Geometry check sheet. Reference: the model listing, model coordinates, mm. A direction names the side the tool comes from. Give positions to 0.01 mm unless a question says otherwise; leave off trailing zeros. Order: outer loops, then holes, each group sorted by start corner. A loop starts at its lowest first (then second) coordinate and runs counter-clockwise, first axis right, second up. Notation, with made-up numbers: M 39,3.25 L 70,3.25 A23 ccw 70,12.25 Z; hole C 5,15.5 d9. An arc over 180 degrees is marked long. Answer as CSV lines item,"result". Start each with the question number.
```python
from build123d import *

# Parameters (mm, degrees)
ESBO_O1_R                = 1.5
ESBO_O1_W                = 15
ESBO_O1_H                = 4
ESBO_O1_W_2              = 5
ESBO_O1_H_2              = 12
RESSALTO_EXTRUS_O1_DEPTH = 5
ESBO_O1_3_W              = 5
ESBO_O1_3_H              = 12
ESBO_O1_3_W_2            = 15
ESBO_O1_3_H_2            = 4
CORTE_EXTRUS_O1_DEPTH    = 2
RESSALTO_EXTRUS_O2_DEPTH = 10
ESBO_O3_R                = 1.5
CORTE_EXTRUS_O2_DEPTH    = 10


with BuildPart() as part:
    # Esbo_o1 → Ressalto-extrus_o1 (new body)
    with BuildSketch(Plane.XY):
        with BuildLine():
            ThreePointArc((40, 3), (39.121320344, 0.878679656), (37, 0))
            Line((37, 0), (0, 0))
            Line((0, 0), (0, 13))
            ThreePointArc((0, 13), (0.878679656, 15.121320344), (3, 16))
            Line((3, 16), (40, 16))
            Line((40, 16), (40, 3))
        make_face()
        with Locations((38, 14)):
            Circle(ESBO_O1_R, mode=Mode.SUBTRACT)
        with Locations((19, 14)):
            Circle(ESBO_O1_R, mode=Mode.SUBTRACT)
        with Locations((28.5, 8)):
            Rectangle(ESBO_O1_W, ESBO_O1_H, mode=Mode.SUBTRACT)
        with Locations((13, 8)):
            Rectangle(ESBO_O1_W_2, ESBO_O1_H_2, mode=Mode.SUBTRACT)
        with Locations((13, 8)):
            Rectangle(ESBO_O1_W_2, ESBO_O1_H_2)
        with Locations((28.5, 8)):
            Rectangle(ESBO_O1_W, ESBO_O1_H)
    extrude(amount=-RESSALTO_EXTRUS_O1_DEPTH)

    # Esbo_o1_3 → Corte-extrus_o1 (cut)
    with BuildSketch(Plane.XY):
        with Locations((13, 8)):
            Rectangle(ESBO_O1_3_W, ESBO_O1_3_H)
        with Locations((28.5, 8)):
            Rectangle(ESBO_O1_3_W_2, ESBO_O1_3_H_2)
    extrude(amount=-CORTE_EXTRUS_O1_DEPTH, mode=Mode.SUBTRACT)

    # Esbo_o2 → Ressalto-extrus_o2 (add)
    with BuildSketch(Plane.XZ):
        with BuildLine():
            Line((19.1, -5), (12.000000019, -5))
            ThreePointArc((12.000000019, -5), (17.086118989, -9.723976561), (12.75, -15.144551516))
            Line((12.75, -15.144551516), (12.75, -21.64580018))
            Line((12.75, -21.64580018), (14.75, -21.64580018))
            Line((14.75, -21.64580018), (14.75, -16.64580018))
            ThreePointArc((14.75, -16.64580018), (17.913332394, -14.029694645), (19.1, -10.1))
            Line((19.1, -10.1), (19.1, -5))
        make_face()
        with BuildLine():
            Line((12.000000019, -5), (4.9, -5))
            Line((4.9, -5), (4.9, -10.1))
            ThreePointArc((4.9, -10.1), (6.086667606, -14.029694645), (9.25, -16.64580018))
            Line((9.25, -16.64580018), (9.25, -21.64580018))
            Line((9.25, -21.64580018), (11.25, -21.64580018))
            Line((11.25, -21.64580018), (11.25, -15.144551516))
            ThreePointArc((11.25, -15.144551516), (6.913881012, -9.723976542), (12.000000019, -5))
        make_face()
    extrude(amount=-RESSALTO_EXTRUS_O2_DEPTH)

    # Esbo_o3 → Corte-extrus_o2 (cut)
    with BuildSketch(Plane(origin=(14.75, 0, 0), x_dir=(0, 0, -1), z_dir=(1, 0, 0))):
        with Locations((19.14580018, 5)):
            Circle(ESBO_O3_R)
    extrude(amount=-CORTE_EXTRUS_O2_DEPTH, mode=Mode.SUBTRACT)


solid = part.part
```
Item 1: Section check C-C on x = 7.5. Record the boundary of the cut face in (y, z).
Item 2: Draft check along Y on faces 5 (the face through (28, 10, -1)), 6 (the face through (36, 8, -1)), 7 (the face through (0, 6, -2)), 8 (the face through (39.14, 0.9, -2.46)). Enter one of: pulls with the +Y half, pulls with the -Y half, needs draft (parallel to the pull), parting line crosses it, or undercut.
Item 3: Access from +Z, -Z, +X, -X, +Y, -Y to the whole of each face (thin tool, end or side, straight path). Record for faces 1 (the face through (4.9, 5, -8)), 2 (the face through (11.25, 6, -17.7)), 3 (the face through (13, 14, -1)), 4 (the face through (7.6, 10, -13.3)).
Item 4: Scan lines: line 1 along Y through (x, z) = (19, -3.5); line 2 along Y through (x, z) = (7, -7.25); line 3 along Z through (x, y) = (24.5, 13.25). Record each from-to range of solid material in increasing order.
Item 5: Depth check by flat-ended pin: pin 1 Ø5 at (x, y) = (31.5, 4.5) entering from -Z; pin 2 Ø5 at (y, z) = (3.5, -18) entering from +X; pin 3 Ø3.5 at (x, z) = (15, -13) entering from +Y. Enter the tip coordinate at first touch or a pass-through.
Item 6: Section check A-A on y = 5. Record the boundary of the cut face in (x, z).
Item 7: Section check D-D on y = 10.75. Record the boundary of the cut face in (x, z), then the cut area to 3 significant figures.
Item 8: Section check B-B on z = -20. Record the boundary of the cut face in (x, y), then the cut area to 3 significant figures.
Numbers:
1,outline,"M 0,-15.59 L 10,-15.59 L 10,-12.5 L 0,-12.5 Z; M 0,-7.7 L 10,-7.7 L 10,-5 L 16,-5 L 16,0 L 0,0 Z"
2,face 5,"undercut"
2,face 6,"undercut"
2,face 7,"needs draft"
2,face 8,"pulls with the -Y half"
3,face 1,"-Z, -X, +Y, -Y"
3,face 2,"-Z, +Y, -Y"
3,face 3,"+Z"
3,face 4,"-Z, +X, -X, +Y"
4,line 1,"0 to 12.5, 15.5 to 16"
4,line 2,"0 to 10"
4,line 3,"-5 to 0"
5,pin 1,"z = -5"
5,pin 2,"x = 16.61"
5,pin 3,"y = 10"
6,outline,"M 0,-5 L 4.9,-5 L 4.9,-10.1 A7.1 ccw 9.25,-16.65 L 9.25,-17.65 L 11.25,-17.65 L 11.25,-15.14 A5.1 cw long 12.75,-15.14 L 12.75,-17.65 L 14.75,-17.65 L 14.75,-16.65 A7.1 ccw 19.1,-10.1 L 19.1,-5 L 40,-5 L 40,0 L 15.5,0 L 15.5,-2 L 10.5,-2 L 10.5,0 L 0,0 Z; M 9.25,-21.65 L 11.25,-21.65 L 11.25,-20.65 L 9.25,-20.65 Z; M 12.75,-21.65 L 14.75,-21.65 L 14.75,-20.65 L 12.75,-20.65 Z"
7,outline,"M 0,-5 L 40,-5 L 40,0 L 15.5,0 L 15.5,-2 L 10.5,-2 L 10.5,0 L 0,0 Z"
7,area,"190 mm2"
8,outline,"M 9.25,0 L 11.25,0 L 11.25,3.77 L 9.25,3.77 Z; M 9.25,6.23 L 11.25,6.23 L 11.25,10 L 9.25,10 Z; M 12.75,0 L 14.75,0 L 14.75,3.77 L 12.75,3.77 Z; M 12.75,6.23 L 14.75,6.23 L 14.75,10 L 12.75,10 Z"
8,area,"30.1 mm2"
